Verification items for the finished model (mm, model axes). A direction names the side the tool comes from. Round coordinates to 2 decimals unless told otherwise and drop trailing zeros. Write each loop counter-clockwise with the first axis right and the second up, starting at its lowest first coordinate (ties: lowest second). Pieces come first, ordered by that corner, then holes. Notation, with made-up numbers: M -14.75,20.25 L 25.25,20.25 A30 ccw 25.25,53.25 Z; hole C 15,68 d1. An arc over 180 degrees is marked long. One line per item, written item: value. Start each with the question number.
Item 1: Gauge pin test, flat ends, axial feed: pin 1 (1 mm diameter, centred on x = -0.5, z = 2.5, fed in from +Y); pin 2 (1 mm diameter, centred on x = 0, z = 0, fed in from -Y). Record the tip position at first contact, or that the pin passes through.
Item 2: Section check A-A, the plane y = 4.25. Record the cut outline in (x, z), then the cut area to 3 significant figures.
Item 3: Tool access check on faces 4 (the face through (-0.7, 10, -1.5)), 5 (the face through (1, 10.6, 0)). Record the directions out of +Z, -Z, +X, -X, +Y, -Y that give a thin tool (end or side, any length) a straight path to the whole face; none if there is none.
Item 4: Draft check along X on faces 1 (the face through (-1.5, 5.07, -0.07)), 2 (the face through (-1, 0, 0)), 3 (the face through (0.323, 5.226, -0.506)). Enter one of: +X half, -X half, draft (parallel to the pull), parting line (faces both ways), or undercut.
Item 5: Thickness scan on probe 1 along X at (y, z) = (3.75, 0); probe 2 along Y at (x, z) = (-0.75, -1.5). Record the ranges inside material, lowest first. Write a range as from..to.
from build123d import *


with BuildPart() as part:
    # Sketch1 → Revolve1 (revolve)
    with BuildSketch(Plane.XY):
        with BuildLine():
            Line((0.6, 0), (1.5, 0))
            Line((1.5, 0), (1.5, 10))
            Line((1.5, 10), (3.2, 10))
            Line((3.2, 10), (3.2, 10.2))
            ThreePointArc((3.2, 10.2), (2.415579075, 10.462316301), (1.6, 10.6))
            Line((1.6, 10.6), (0.6, 10.6))
            Line((0.6, 10.6), (0.6, 0))
        make_face()
    revolve(axis=Axis((0, 0, 0), (0, 1, 0)))


solid = part.part
Response values:
1. pin 1: stops at y = 10.54
1. pin 2: passes through
2. outline: C 0,0 d3; hole C 0,0 d1.2
2. area: 5.94 mm2
3. face 4: -Y
3. face 5: +Z, -Z, +X, -X, +Y
4. face 1: parting line
4. face 2: draft
4. face 3: undercut
5. probe 1: x = -1.5..-0.6, 0.6..1.5
5. probe 2: y = 10..10.59
